```python
from build123d import *

# Parameters (mm, degrees)
BASE_R_VOLUTION_ANGLE   = 180
ESQUISSE2_W             = 44
ESQUISSE2_H             = 6
ENL_V_MAT_EXTRU_1_DEPTH = 25


with BuildPart() as part:
    # Esquisse1 → Base-Révolution (revolve, symmetric)
    with BuildSketch(Plane.XY) as base_r_volution_sk:
        with BuildLine():
            Line((-12, 17.839562775), (-12, 24))
            ThreePointArc((-12, 24), (-11.414213562, 25.414213562), (-10, 26))
            Line((-10, 26), (10, 26))
            ThreePointArc((10, 26), (11.414213562, 25.414213562), (12, 24))
            Line((12, 24), (12, 17.839562775))
            ThreePointArc((12, 17.839562775), (0, 21.5), (-12, 17.839562775))
        make_face()
    revolve(axis=Axis((-22, 0, 0), (1, 0, 0)), revolution_arc=BASE_R_VOLUTION_ANGLE / 2)
    revolve(base_r_volution_sk.sketch, axis=Axis((-22, 0, 0), (-1, 0, 0)), revolution_arc=BASE_R_VOLUTION_ANGLE / 2)

    # Esquisse2 → Enlèv. mat.-Extru.1 (cut, through all)
    with BuildSketch(Plane(origin=(12, 0, 0), x_dir=(0, 0, -1), z_dir=(1, 0, 0))):
        with Locations((0, 27)):
            Rectangle(ESQUISSE2_W, ESQUISSE2_H)
    extrude(amount=-ENL_V_MAT_EXTRU_1_DEPTH, mode=Mode.SUBTRACT)


solid = part.part
```
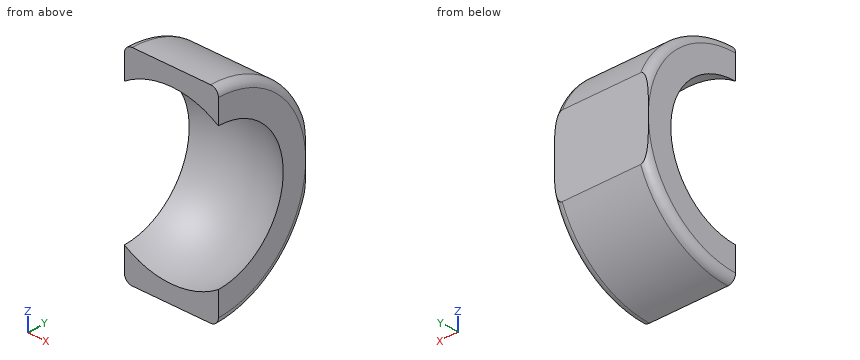
The model under review builds one solid part; all positions refer to its coordinate system, in mm. Coordinates: 2 decimals unless noted, no trailing zeros. Write each loop counter-clockwise with the first axis right and the second up, starting at its lowest first coordinate (ties: lowest second). Pieces come first, ordered by that corner, then holes. Notation, with made-up numbers: (-1, 25.25) - (51, 25.25) arc R16 cw to (51, 37.25) - close; hole circle Ø8 at (-30, 54.5). An arc over 180 degrees is marked (long way). Write item = value, one per line.
(1) For P1, Ø1.5, axis at x = -2.5, y = 9, coming from the +Z side; P2, Ø2, axis at x = 3.5, z = 17, coming from the -Y side; P3, Ø1.5, axis at x = -7, y = 13, coming from the -Z side, all flat-tipped, find the tip position at first contact; note any pin that passes through.
Result sheet:
P1 = 24.66
P2 = 11.19
P3 = -22.93
(2) For line 1 (Z direction, x = -9.25, y = 6.5); line 2 (Z direction, x = 0.25, y = 8.25); line 3 (Y direction, x = 11.25, z = -5), list the stretches that pass through material, from the lowest coordinate up. Write a range as [from, to].
Result sheet:
line_1 = [-25.17, -18.29], [18.29, 25.17]
line_2 = [-24.66, -19.85], [19.85, 24.66]
line_3 = [17.63, 24]
(3) Consider section A-A, the plane x = 0.5. Give the boundary of the cut face in (y, z).
Result sheet:
outline = (0, -26) arc R26 ccw to (24, -10) - (24, 10) arc R26 ccw to (0, 26) - (0, 21.49) arc R21.49 cw to (0, -21.49) - close
(4) Consider section B-B, the plane x = -5.75. Give the boundary of the cut face in (y, z), then the cut area to 3 significant figures.
Result sheet:
outline = (0, -26) arc R26 ccw to (24, -10) - (24, 10) arc R26 ccw to (0, 26) - (0, 20.72) arc R20.72 cw to (0, -20.72) - close
area = 361 mm^2
